Can you work these out from the model? Positions are in its coordinate system, mm. A direction names the side the tool comes from. Round coordinates to 2 decimals unless told otherwise and drop trailing zeros. Order: outer loops, then holes, each group sorted by start corner. A loop starts at its lowest first (then second) coordinate and runs counter-clockwise, first axis right, second up. Notation, with made-up numbers: M 49,13 L 60,13 A12 ccw 60,18 Z; hole C -39.5,76 d8. An arc over 180 degrees is marked long. One line per question, with ' | ' between items.
```python
from build123d import *

# Parameters (mm, degrees)
CHAMFER1_SIZE      = 3.81
CHAMFER1_SIZE2     = 0.671805796
FILLET2_R          = 0.508
FILLET3_R          = 38.1
CHAMFER2_SIZE      = 0.762
CHAMFER2_SIZE2     = 0.135060614
FILLET4_R          = 0.254
SKETCH6_R          = 2.950428165
CUT_EXTRUDE1_DEPTH = 28.612445783
FILLET5_R          = 2.54


with BuildPart() as part:
    # Sketch3 → Revolve1 (revolve)
    with BuildSketch(Plane(origin=(0, 0, 0), x_dir=(0, 0, -1), z_dir=(1, 0, 0))):
        with BuildLine():
            Line((-3.331428165, 0.1905), (-2.950428165, -13.7795))
            Line((-2.950428165, -13.7795), (-2.950428165, -22.6695))
            Line((-2.950428165, -22.6695), (0, -22.6695))
            Line((0, -22.6695), (0, -24.1935))
            add(Edge.make_bspline(
                [(-10.951428165, -22.6695), (-7.67361224, -23.87858079), (-8.424695912, -25.057739032), (-3.760861411, -24.039674634), (-1.096246091, -24.1935), (0, -24.1935)],
                knots=[0, 0, 0, 0, 0.345230168, 0.440287605, 1, 1, 1, 1], degree=3))
            Line((-10.951428165, -22.6695), (-5.871428165, -22.6695))
            Line((-5.871428165, -22.6695), (-5.871428165, 0.1905))
            Line((-5.871428165, 0.1905), (-3.331428165, 0.1905))
        make_face()
    revolve(axis=Axis((0, -22.6695, 0), (0, -1, 0)))

    # Chamfer1
    chamfer1_edges = [part.edges().sort_by_distance(p)[0] for p in [
        (0, 0.1905, -5.871428165),
    ]]
    chamfer1_side = [part.faces().sort_by_distance(p)[0] for p in [
        (0, -11.2395, -5.871428165),
    ]]
    chamfer(chamfer1_edges, length=CHAMFER1_SIZE, length2=CHAMFER1_SIZE2, reference=chamfer1_side[0])

    # Fillet2
    fillet2_edges = [part.edges().sort_by_distance(p)[0] for p in [
        (0, 0.1905, -5.199622369),
    ]]
    fillet(fillet2_edges, radius=FILLET2_R)

    # Fillet3
    fillet3_edges = [part.edges().sort_by_distance(p)[0] for p in [
        (0, -3.6195, -5.871428165),
    ]]
    fillet(fillet3_edges, radius=FILLET3_R)

    # Chamfer2
    chamfer2_edges = [part.edges().sort_by_distance(p)[0] for p in [
        (0, 0.1905, -3.331428165),
    ]]
    chamfer2_side = [part.faces().sort_by_distance(p)[0] for p in [
        (0, -6.7945, -3.140928165),
    ]]
    chamfer(chamfer2_edges, length=CHAMFER2_SIZE, length2=CHAMFER2_SIZE2, reference=chamfer2_side[0])

    # Fillet4
    fillet4_edges = [part.edges().sort_by_distance(p)[0] for p in [
        (0, 0.1905, -3.46648878),
    ]]
    fillet(fillet4_edges, radius=FILLET4_R)

    # Sketch6 → Cut-Extrude1 (cut, through all)
    with BuildSketch(Plane(origin=(0, -22.6695, 0), x_dir=(1, 0, 0), z_dir=(0, 1, 0))):
        with Locations(Location((0, 0, 0), (0, 0, 270))):
            Circle(SKETCH6_R)
    extrude(amount=-CUT_EXTRUDE1_DEPTH, mode=Mode.SUBTRACT)

    # Fillet5
    fillet5_edges = [part.edges().sort_by_distance(p)[0] for p in [
        (2e-09, -24.204539733, -2.950428166),
    ]]
    fillet(fillet5_edges, radius=FILLET5_R)


solid = part.part
```
(1) Will these pins go through, and if not, where does the flat tip stop? pin 1 Ø1.5 at (y, z) = (-3.5, -0.5) entering from -X; pin 2 Ø6 at (y, z) = (-8, 3.5) entering from +X; pin 3 Ø3 at (y, z) = (-15, 4.5) entering from -X.
Final values:
pin 1: x = -5.77 | pin 2: x = 5.85 | pin 3: x = -5.05
(2) On a 3-axis mill with a long thin cutter (end or side, diameter ignored), from which of +Z, -Z, +X, -X, +Y, -Y can I reach the whole of each face in a straight line? I mean faces 1 (the flat face through (5, -22.67, 5)), 2 (the cylindrical face through (1.13, -17.889, 2.725)). Say none if no direction works.
Final values:
face 1: +Y | face 2: +Y, -Y
(3) If we section it at B-B on y = -9: Please give me the cut outline in (x, z), plus the area to 3 significant figures.
Final values:
outline: C 0,0 d11.74; hole C 0,0 d6.16 | area: 78.5 mm^2
(4) Please list where these lines run through material, in increasing order: probe 1 along Z at (x, y) = (0, -19.75); probe 2 along Z at (x, y) = (2, -2). Write a range as [from, to].
Final values:
probe 1: [-5.87, -2.95], [2.95, 5.87] | probe 2: [-5.18, -2.59], [2.59, 5.18]
(5) If we section it at A-A on y = -15: Please give me the cut outline in (x, z).
Final values:
outline: C 0,0 d11.74; hole C 0,0 d5.9
(6) Thinking about a two-plate mould opening in X: for faces 3 (the cylindrical face through (-1.76, -14.7, 5.6)), 4 (the flat face through (4, 0.191, 1)), 5 (the conical face through (1.903, -7.268, -2.482)), which applies, released by +X, released by -X, zero draft, split by the parting line, or undercut?
Final values:
face 3: split by the parting line | face 4: zero draft | face 5: undercut
